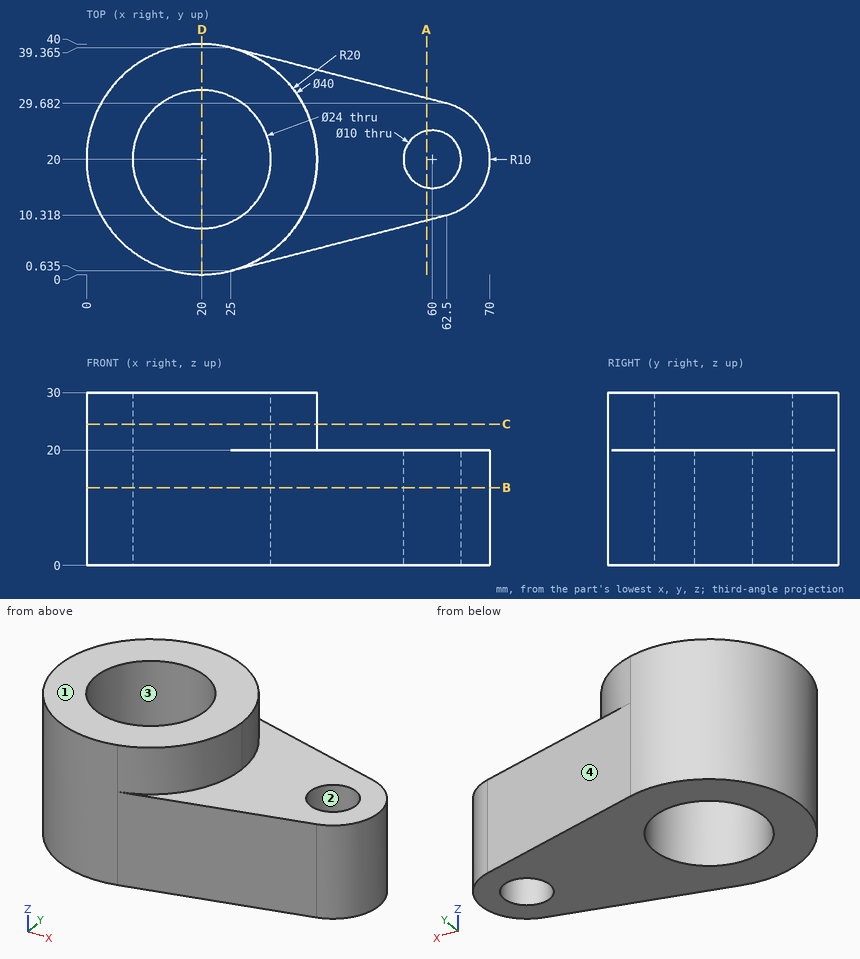
The figure shows three views and two pictorial views of one solid part (mm, origin at its lowest corner). Answer the questions. Coordinates: 2 decimals unless noted, no trailing zeros. Order: outer loops, then holes, each group sorted by start corner. A loop starts at its lowest first (then second) coordinate and runs counter-clockwise, first axis right, second up. Notation, with made-up numbers: (-27, -11.75) - (-20, -11.75) arc R24 ccw to (-20, 3.25) - close; hole circle Ø9 at (77, 55). An arc over 180 degrees is marked (long way). Answer as a JSON object with one key per item and string values.
1. Find section B-B on z = 13.5. Determine the outline of the cut face in (x, y) (1 decimal).
Output values:
{"outline": "(25, 0.6) - (62.5, 10.3) arc R10 ccw to (62.5, 29.7) - (25, 39.4) arc R20 ccw (long way) to start; hole circle Ø24 at (20, 20); hole circle Ø10 at (60, 20)"}
2. Find section C-C on z = 24.5. Determine the outline of the cut face in (x, y) (1 decimal), plus the area to 3 significant figures.
Output values:
{"outline": "(25, 0.6) arc R20 ccw to (25, 39.4) arc R20 ccw (long way) to start; hole circle Ø24 at (20, 20)", "area": "804 mm²"}
3. Each of these flat-tipped pins is pushed along its axis until it touches: P1, Ø9, axis at x = 60, y = 20, coming from the +Z side; P2, Ø4, axis at x = 45.5, y = 13, coming from the -Z side; P3, Ø4, axis at x = 33.5, z = 16.5, coming from the +Y side; P4, Ø5, axis at x = 38, z = 6.5, coming from the +Y side. Where does it stop, or does it pass through?
Output values:
{"P1": "passes through", "P2": "stops at z = 0", "P3": "stops at y = 37.69", "P4": "stops at y = 36.65"}
4. Find section A-A on x = 59. Determine the outline of the cut face in (y, z).
Output values:
{"outline": "(9.41, 0) - (15.1, 0) - (15.1, 20) - (9.41, 20) - close; (24.9, 0) - (30.59, 0) - (30.59, 20) - (24.9, 20) - close"}
5. The mould has two halves that part along X. Classify the marked faces 1, 2, 3 and 4: +X half, -X half, draft (parallel to the pull), parting line (faces both ways), or undercut.
Output values:
{"face 1": "draft", "face 2": "undercut", "face 3": "undercut", "face 4": "+X half"}
6. Find section D-D on x = 20. Determine the outline of the cut face in (y, z), plus the area to 3 significant figures.
Output values:
{"outline": "(0, 0) - (8, 0) - (8, 30) - (0, 30) - close; (32, 0) - (40, 0) - (40, 30) - (32, 30) - close", "area": "480 mm²"}
7. Consider line 1 (Y direction, x = 20, z = 15.5); line 2 (Z direction, x = 65.5, y = 21); line 3 (Y direction, x = 30, z = 17.5) (1 decimal). Determine where each line is inside the solid, lowest interval first.
Output values:
{"line 1": "y = 0 to 8, 32 to 40", "line 2": "z = 0 to 20", "line 3": "y = 1.9 to 13.4, 26.6 to 38.1"}
